from build123d import *

# Parameters (mm, degrees)
BOSS_EXTRUDE1_DEPTH = 3
SKETCH2_W           = 60
SKETCH2_H           = 2.5
BOSS_EXTRUDE2_DEPTH = 40
SKETCH5_W           = 60
SKETCH5_H           = 1.359629359
BOSS_EXTRUDE5_DEPTH = 57.5
FILLET1_R           = 10
SKETCH6_W           = 2
SKETCH6_H           = 102.169483657
BOSS_EXTRUDE6_DEPTH = 20


with BuildPart() as part:
    # Sketch1 → Boss-Extrude1 (new body)
    with BuildSketch(Plane(origin=(0, 0, 0), x_dir=(1, 0, 0), z_dir=(0, 1, 0))):
        Polygon((106.407471576, 20), (207.407471576, 20), (207.407471576, 0), (250, 0), (250, 24.022028172), (176.397365129, 24.022028172), (176.397365129, 126.191511829), (250, 126.191511829), (250, 150), (207.407471576, 150), (207.407471576, 130), (106.407471576, 130), (106.407471576, 150), (0, 150), (0, 0), (106.407471576, 0), align=None)
    extrude(amount=BOSS_EXTRUDE1_DEPTH)

    # Sketch2 → Boss-Extrude2 (add)
    with BuildSketch(Plane(origin=(0, 3, 0), x_dir=(1, 0, 0), z_dir=(0, 1, 0))):
        with Locations((69.460984605, 106.25)):
            Rectangle(SKETCH2_W, SKETCH2_H)
        with Locations((69.460984605, 46.25)):
            Rectangle(SKETCH2_W, SKETCH2_H)
    extrude(amount=BOSS_EXTRUDE2_DEPTH)

    # Sketch5 → Boss-Extrude5 (add)
    with BuildSketch(Plane(origin=(0, 0, -47.5), x_dir=(-1, 0, 0), z_dir=(0, 0, -1))):
        with Locations((-69.460984605, 42.320185321)):
            Rectangle(SKETCH5_W, SKETCH5_H)
    extrude(amount=BOSS_EXTRUDE5_DEPTH)

    # Fillet1
    fillet1_edges = [part.edges().sort_by_distance(p)[0] for p in [
        (0, 1.5, -150),
        (250, 1.5, -150),
        (250, 1.5, 0),
        (0, 1.5, 0),
    ]]
    fillet(fillet1_edges, radius=FILLET1_R)

    # Sketch6 → Boss-Extrude6 (add)
    with BuildSketch(Plane(origin=(0, 3, 0), x_dir=(1, 0, 0), z_dir=(0, 1, 0))):
        with Locations((175.397365129, 75.106770001)):
            Rectangle(SKETCH6_W, SKETCH6_H)
    extrude(amount=BOSS_EXTRUDE6_DEPTH)


solid = part.part
Can you work these out from the model? Positions are in its coordinate system, mm. A direction names the side the tool comes from. Coordinates: 2 decimals unless noted, no trailing zeros. Write each loop counter-clockwise with the first axis right and the second up, starting at its lowest first coordinate (ties: lowest second). Pieces come first, ordered by that corner, then holes.
Q1. Imagine slicing it at C-C, the plane y = 17. List the corners of the cut face in (x, z) for me, plus the area to 3 significant figures.
Results found:
outline: (39.46, -107.5) - (99.46, -107.5) - (99.46, -105) - (39.46, -105) - close; (39.46, -47.5) - (99.46, -47.5) - (99.46, -45) - (39.46, -45) - close; (174.4, -126.19) - (176.4, -126.19) - (176.4, -24.02) - (174.4, -24.02) - close
area: 504 mm2
Q2. Which directions (+Z, -Z, +X, -X, +Y, -Y) give clear straight access to the entire face, cutting with the end or side of a thin tool? Please do faces 1 (the face through (69, 23, -45)), 2 (the face through (69, 23, -107.5)), 3 (the face through (69, 22, -47.5)).
Results found:
face 1: +Z, -X, +Y
face 2: -Z, -X, +Y
face 3: -X
Q3. Please list where these lines run through material, in increasing order: L1, parallel to Y at x = 67, z = -103; L2, parallel to Z at x = 77, y = 21; L3, parallel to Y at x = 29.5, z = -70.
Results found:
L1: y = 0 to 3, 41.64 to 43
L2: z = -107.5 to -105, -47.5 to -45
L3: y = 0 to 3
Q4. For P1, Ø5, axis at x = 114.5, z = -56, coming from the -Y side; P2, Ø5, axis at x = 103, z = -16, coming from the +Y side; P3, Ø5, axis at y = 19.5, z = -56, coming from the -X side; P4, Ø7, axis at y = 16, z = -97.5, coming from the +X side, each with a flat end and sliding along its axis, tell me the tip position at first contact or that it passes through.
Results found:
P1: stops at y = 0
P2: stops at y = 3
P3: stops at x = 174.4
P4: stops at x = 176.4
Q5. Imagine slicing it at B-B, the plane x = 45. List the corners of the cut face in (y, z) for me.
Results found:
outline: (0, -150) - (3, -150) - (3, -107.5) - (43, -107.5) - (43, -45) - (3, -45) - (3, 0) - (0, 0) - close; hole (3, -105) - (41.64, -105) - (41.64, -47.5) - (3, -47.5) - close
Q6. If we mould it in two halves opening along Y, with no side actions, what happens to faces 4 (the face through (70, 41.64, -76)), 5 (the face through (69, 22, -105)), 6 (the face through (95, 0, -76)), 7 (the face through (176.397, 11, -74))? For each: +Y half, -Y half, draft (parallel to the pull), parting line (faces both ways), or undercut.
Results found:
face 4: undercut
face 5: undercut
face 6: -Y half
face 7: draft
Q7. Imagine slicing it at A-A, the plane y = 28.5. List the corners of the cut face in (x, z) for me.
Results found:
outline: (39.46, -107.5) - (99.46, -107.5) - (99.46, -105) - (39.46, -105) - close; (39.46, -47.5) - (99.46, -47.5) - (99.46, -45) - (39.46, -45) - close
Q8. Imagine slicing it at D-D, the plane z = -16. List the corners of the cut face in (x, y) for me.
Results found:
outline: (0, 0) - (106.41, 0) - (106.41, 3) - (0, 3) - close; (207.41, 0) - (250, 0) - (250, 3) - (207.41, 3) - close
